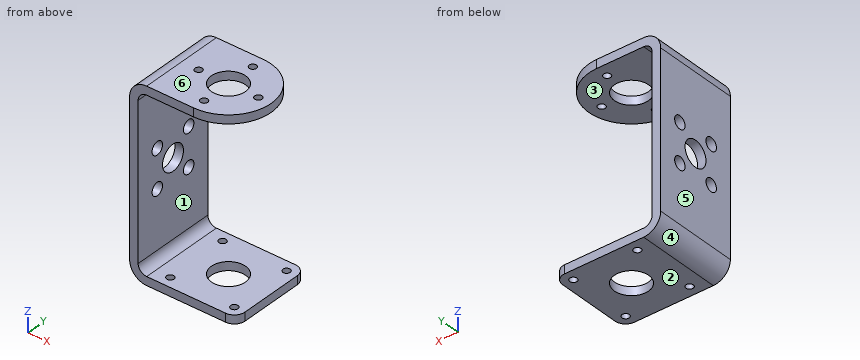
Autodesk Inventor part; units mm, degrees
ref_plane "YZ Plane" through (0, 0, 0) normal (1, 0, 0) x (0, 1, 0)
ref_plane "XZ Plane" through (0, 0, 0) normal (0, 1, 0) x (-1, 0, 0)
ref_plane "XY Plane" through (0, 0, 0) normal (0, 0, 1) x (1, 0, 0)
sketch "Sketch1" plane through (0, 0, 0) normal (0, 0, 1) x (1, 0, 0)
  line L0 (2.5, 10) -> (37.5, 10) construction
  line L1 (0, -7.5) -> (0, 7.5) construction
  line L2 (37.5, -10) -> (2.5, -10) construction
  circle A0 centre (10, -7) radius 0.85
  circle A1 centre (10, 7) radius 0.85
  circle A2 centre (3, 0) radius 0.85
  circle A3 centre (10, 0) radius 10
  line L3 (10, 7) -> (10, -7) construction
  circle A4 centre (17, 0) radius 0.85
  line L4 (10, 10) -> (-5, 10)
  line L5 (-5, 10) -> (-5, -10)
  line L6 (-5, -10) -> (10, -10)
  line L7 (10, -10) -> (10, 10)
  line L8 (10, 0) -> (20, 0)
  point P0 (0, 0)
  dimension "d0" = 25
extrude "Plate1" add sketch "Sketch1" along normal blind 2 contours A0 L7 L8 A4 A3 | A0 L7 A3 A1 | L7 A1 A3 L8 A4 | L6 L5 L4 A3
sketch "Sketch2" plane through (-3, 10, 2) normal (-1, 0, 0) x (0, -1, 0)
  line L0 (20, 0) -> (0, 0)
  line L1 (0, 0) -> (0, -44)
  line L2 (0, -44) -> (20, -44)
  line L3 (20, -44) -> (20, 0)
edge flange "Flange1" height 44 angle 90 thickness 2 bend radius 2 thickness toward (-1, 0, 0) relief tear relief width 2 relief depth 1 edges at (-5, 0, 0) wall of the first edge with corners at (-3, -10, 2) (-3, 10, 2) (-3, 10, -42) (-3, -10, -42)
bend "Bend1"
corner "Corner1"
sketch "Sketch3" plane through (-5, 10, -40) normal (0, 0, -1) x (-1, 0, 0)
  line L0 (0, -20) -> (0, 0)
  line L1 (0, 0) -> (-25, 0)
  line L2 (-25, 0) -> (-25, -20)
  line L3 (-25, -20) -> (0, -20)
edge flange "Flange2" height 25 angle 90 thickness 2 bend radius 2 thickness toward (0, 0, -1) relief tear relief width 2 relief depth 1 edges at (-3, 0, -42) wall of the first edge with corners at (-5, -10, -40) (-5, 10, -40) (20, 10, -40) (20, -10, -40)
bend "Bend2"
corner "Corner2"
fillet "Fillet1" radius 2.5 2 edges at (20, 10, -41) (20, -10, -41)
sketch "Sketch4" plane through (-1, -10, -42) normal (0, 0, -1) x (-1, 0, 0)
  circle A0 centre (-18.5, 2.5) radius 0.85
  circle A1 centre (-18.5, 17.5) radius 0.85
  circle A2 centre (-3.5, 17.5) radius 0.85
  circle A3 centre (-3.5, 2.5) radius 0.85
  point P0 (-1, 10)
extrude "Cut1" cut sketch "Sketch4" against normal blind 2
sketch "Sketch5" plane through (-5, -10, -2) normal (-1, 0, 0) x (0, 0, 1)
  line L0 (-36, 20) -> (0, 20) construction
  line L1 (-18, 20) -> (-18, 0) construction
  line L2 (0, 0) -> (-36, 0) construction
  circle A0 centre (-18, 10) radius 3
  line L3 (-22.5, 14.5) -> (-13.5, 14.5) construction
  line L4 (-13.5, 14.5) -> (-13.5, 5.5) construction
  line L5 (-13.5, 5.5) -> (-22.5, 5.5) construction
  line L6 (-22.5, 5.5) -> (-22.5, 14.5) construction
  line L7 (-22.5, 14.5) -> (-13.5, 5.5) construction
  circle A1 centre (-13.5, 14.5) radius 1.5
  circle A2 centre (-22.5, 14.5) radius 1.5
  circle A3 centre (-22.5, 5.5) radius 1.5
  circle A4 centre (-13.5, 5.5) radius 1.5
  point P0 (2, 10)
  dimension "d25" = 6
  dimension "d26" = 9
  dimension "d27" = 3
extrude "Cut2" cut sketch "Sketch5" against normal blind 2
sketch "Sketch6" plane through (0, 0, 2) normal (0, 0, 1) x (1, 0, 0)
  arc A0 (10, -10) -> (10, 10) centre (10, 0) ccw construction
  circle A1 centre (10, 0) radius 4
  point P0 (0, 0)
  dimension "d30" = 8
extrude "Cut3" cut sketch "Sketch6" against normal through all
equation "\"d23\" = Thickness"
equation "\"d28\" = Thickness"
equation "\"d31\" = Thickness"
equation "\"d1\" = Thickness"
equation "\"d2\" = BendReliefWidth"
equation "\"d3\" = BendReliefDepth"
equation "\"d4\" = MinimumRemnant"
equation "\"d5\" = TransitionRadius"
equation "\"d8\" = BendRadius"
equation "\"d9\" = CornerReliefSize"
equation "\"d10\" = GapSize"
equation "\"d11\" = JacobiRadiusSize"
equation "\"d12\" = BendReliefWidth"
equation "\"d13\" = BendReliefDepth"
equation "\"d14\" = MinimumRemnant"
equation "\"d15\" = TransitionRadius"
equation "\"d18\" = BendRadius"
equation "\"d19\" = CornerReliefSize"
equation "\"d20\" = GapSize"
equation "\"d21\" = JacobiRadiusSize"
equation "\"BendRadius\" = Thickness"
equation "\"BendReliefWidth\" = Thickness"
equation "\"BendReliefDepth\" = 0.5 * Thickness"
equation "\"CornerReliefSize\" = 4 * Thickness"
equation "\"MinimumRemnant\" = 2 * Thickness"
equation "\"TransitionRadius\" = BendRadius"
equation "\"JacobiRadiusSize\" = BendRadius"
equation "\"GapSize\" = Thickness"
Can you work these out from the model? Positions are in its coordinate system, mm. Face numbers are marked on the shaded views. A direction names the side the tool comes from. Coordinates: 2 decimals unless noted, no trailing zeros. Order: outer loops, then holes, each group sorted by start corner. A loop starts at its lowest first (then second) coordinate and runs counter-clockwise, first axis right, second up. Notation, with made-up numbers: (29.25, 27) -> (39.25, 27) arc R6 ccw to (39.25, 33) -> close; hole circle Ø8 at (60, 49.5). An arc over 180 degrees is marked (long way). Write each question's results on one line, items separated by ' | '.
Item 1: Which directions (+Z, -Z, +X, -X, +Y, -Y) give clear straight access to the entire face, cutting with the end or side of a thin tool? Please do the marked faces 1 and 2.
Results are:
face 1: +X, +Y, -Y | face 2: -Z, +X, -X, +Y, -Y
Item 2: I want a section at B-B, the plane y = 0. Count the separate pieces of the cut face and the enclosed holes in it, then the cut area to 3 significant figures.
Results are:
separate pieces: 6 | enclosed holes: 0 | area: 124 mm²
Item 3: I want a section at C-C, the plane x = -0.25. Write out the boundary of the cut face in (y, z).
Results are:
outline: (-10, -42) -> (10, -42) -> (10, -40) -> (-10, -40) -> close; (-10, 0) -> (10, 0) -> (10, 2) -> (-10, 2) -> close
Item 4: If we mould it in two halves opening along Z, with no side actions, what happens to the marked faces 3, 4, 5 and 6? For each: +Z half, -Z half, draft (parallel to the pull), parting line (faces both ways), or undercut.
Results are:
face 3: undercut | face 4: -Z half | face 5: draft | face 6: +Z half
Item 5: I'm going to push flat-ended pins straight in: pin 1 Ø2 at (x, y) = (10, 7) entering from +Z; pin 2 Ø1.4 at (x, y) = (17.5, 7.5) entering from -Z; pin 3 Ø5 at (y, z) = (4, -12.5) entering from +X. Where does each tip first touch, or does it pass through?
Results are:
pin 1: z = 2 | pin 2: z = 0 | pin 3: x = -3
Item 6: I want a section at A-A, the plane z = -20. Write out the boundary of the cut face in (x, y).
Results are:
outline: (-5, -10) -> (-3, -10) -> (-3, -3) -> (-5, -3) -> close; (-5, 3) -> (-3, 3) -> (-3, 10) -> (-5, 10) -> close
Item 7: I want a section at D-D, the plane z = -15.5. Write out the boundary of the cut face in (x, y).
Results are:
outline: (-5, -10) -> (-3, -10) -> (-3, -6) -> (-5, -6) -> close; (-5, -3) -> (-3, -3) -> (-3, 3) -> (-5, 3) -> close; (-5, 6) -> (-3, 6) -> (-3, 10) -> (-5, 10) -> close
Item 8: If I drill on line 1 along Y through (x, z) = (17.5, -40.8); line 2 along Y through (x, z) = (10, 0.55); line 3 along Y through (x, z) = (-4.15, -24.5), over which ranges is the centre line in solid material (lowest first)?
Results are:
line 1: -10 to -8.35, -6.65 to 6.65, 8.35 to 10 | line 2: -10 to -7.85, -6.15 to -4, 4 to 6.15, 7.85 to 10 | line 3: -10 to -6, -3 to 3, 6 to 10
